```python
from build123d import *

# Parameters (mm, degrees)
SKETCH1_R           = 10
BOSS_EXTRUDE1_DEPTH = 5
BOSS_EXTRUDE2_DEPTH = 5
SKETCH3_R           = 12.5
BOSS_EXTRUDE3_DEPTH = 5
SKETCH5_R           = 7.5
BOSS_EXTRUDE4_DEPTH = 5
BOSS_EXTRUDE4_TAPER = 52
CUT_EXTRUDE4_DEPTH  = 26
SKETCH12_R          = 1.5
CUT_EXTRUDE5_DEPTH  = 10


with BuildPart() as part:
    # Sketch1 → Boss-Extrude1 (new body)
    with BuildSketch(Plane.XY):
        Circle(SKETCH1_R)
    extrude(amount=BOSS_EXTRUDE1_DEPTH)

    # Sketch2 → Boss-Extrude2 (add)
    with BuildSketch(Plane(origin=(0, 0, 0), x_dir=(-1, 0, 0), z_dir=(0, 0, -1))):
        with BuildLine():
            Line((28.226697949, 15.611392499), (31.387852607, 23.606970284))
            Line((31.387852607, 23.606970284), (28.492660152, 23.606970284))
            add(Edge.make_bspline(
                [(1.702274754, -2.039901693), (1.751506914, -1.119618262), (1.905629401, 0.736300837), (2.439985578, 4.279152464), (3.573593312, 8.507619636), (5.826230301, 13.181920176), (9.085989857, 17.262755922), (13.259055966, 20.42976386), (18.030055154, 22.500703416), (22.280120083, 23.371095334), (25.78433669, 23.636661982), (27.595284541, 23.636820284), (28.492660152, 23.606970284)],
                knots=[0, 0, 0, 0, 0.0625, 0.125, 0.25, 0.375, 0.5, 0.625, 0.75, 0.875, 0.9375, 1, 1, 1, 1], degree=3))
            Line((1.702274754, -2.039901693), (9.690851664, -2.467264483))
            add(Edge.make_bspline(
                [(9.690851664, -2.467264483), (10.68920872, 16.194753627), (28.226697949, 15.611392499)],
                knots=[0, 0, 0, 1, 1, 1], degree=2))
        make_face()
    extrude(amount=-BOSS_EXTRUDE2_DEPTH)

    # Sketch3 → Boss-Extrude3 (add)
    with BuildSketch(Plane(origin=(-19.073171032, -7.540823824, 0), x_dir=(0, 0, 1), z_dir=(-0.9299562551595503, -0.3676701830304238, 0))):
        with Locations(Location((2.5, 29.194927251, 0), (0, 0, 270))):
            Circle(SKETCH3_R)
    extrude(amount=BOSS_EXTRUDE3_DEPTH)

    # Sketch5 → Boss-Extrude4 (add)
    with BuildSketch(Plane(origin=(-19.073171032, -7.540823824, 0), x_dir=(0, 0, -1), z_dir=(0.9299562551595503, 0.3676701830304238, 0))):
        with Locations((-2.5, 29.194927251)):
            Circle(SKETCH5_R)
    extrude(amount=BOSS_EXTRUDE4_DEPTH, taper=BOSS_EXTRUDE4_TAPER)

    # Sketch11 → Cut-Extrude4 (cut)
    with BuildSketch(Plane.XY.offset(15)):
        Polygon((-39.052933842, 29.395283666), (-26.628493881, 7.42446109), (-33.620316113, 1.865469744), align=None)
    extrude(amount=-CUT_EXTRUDE4_DEPTH, mode=Mode.SUBTRACT)

    # Sketch12 → Cut-Extrude5 (cut)
    with BuildSketch(Plane(origin=(0, 0, 0), x_dir=(-1, 0, 0), z_dir=(0, 0, -1))):
        Circle(SKETCH12_R)
    extrude(amount=-CUT_EXTRUDE5_DEPTH, mode=Mode.SUBTRACT)


solid = part.part
```
CAD build for the part. Positions are in the model's coordinates, mm. Round coordinates to 2 decimals unless told otherwise and drop trailing zeros. Order: outer loops, then holes, each group sorted by start corner. A loop starts at its lowest first (then second) coordinate and runs counter-clockwise, first axis right, second up.
Q1. Slice it at A-A (x = 0). Write the cut outline in (y, z).
Q2. Drop flat-ended pins along their axis: pin 1 (2 mm diameter, centred on y = 18, z = 0.5, fed in from -X); pin 2 (6 mm diameter, centred on x = -6.5, y = 3, fed in from -Z); pin 3 (6 mm diameter, centred on x = 0, z = -2, fed in from +Y). Give the stop position or say it passes through.
Q3. Wall check: L1, parallel to Y at x = 0, z = 3.45; L2, parallel to Z at x = 1, y = -6.5; L3, parallel to X at y = -1, z = 4.25. Give the ranges that are in metal, low to high.
Q4. Two-plate mould, pull along Y, no slides. Class faces 1 (the cylindrical face through (1.5, 0.07, 2.46)), 2 (the flat face through (-32.928, 18.564, 2.675)), 3 (the cylindrical face through (-36.17, 30.52, 3.05)): pulls with the +Y half, pulls with the -Y half, needs draft (parallel to the pull), parting line crosses it, or undercut.
Q5. Slice it at D-D (z = 13.25). Write the cut outline in (x, y).
Q6. Slice it at C-C (y = -6). Write the cut outline in (x, z).
Results below:
1. outline: (-10, 0) - (-1.5, 0) - (-1.5, 5) - (-10, 5) - close; (1.5, 0) - (10, 0) - (10, 5) - (1.5, 5) - close
2. pin 1: stops at x = -33.17
2. pin 2: stops at z = 0
2. pin 3: stops at y = 10
3. L1: y = -10 to -1.5, 1.5 to 10
3. L2: z = 0 to 5
3. L3: x = -9.95 to -1.12, 1.12 to 9.95
4. face 1: undercut
4. face 2: pulls with the -Y half
4. face 3: parting line crosses it
5. outline: (-36.01, 24.02) - (-29.67, 12.8) - (-27.46, 13.68) - (-32.15, 25.54) - close
6. outline: (-8, 0) - (8, 0) - (8, 5) - (-8, 5) - close
